Autodesk Inventor part; units mm, degrees
ref_plane "YZ Plane" through (0, 0, 0) normal (1, 0, 0) x (0, 1, 0)
ref_plane "XZ Plane" through (0, 0, 0) normal (0, 1, 0) x (-1, 0, 0)
ref_plane "XY Plane" through (0, 0, 0) normal (0, 0, 1) x (1, 0, 0)
sketch "Sketch1" plane through (0, 0, 0) normal (0, 0, 1) x (1, 0, 0)
  circle A0 centre (0, 0) radius 20
  line L0 (-85, -85) -> (85, -85)
  line L1 (85, -85) -> (85, 85)
  line L2 (85, 85) -> (-85, 85)
  line L3 (-85, 85) -> (-85, -85)
  line L4 (-85, -85) -> (85, 85) construction
  line L5 (85, -85) -> (-85, 85) construction
  dimension "d0" = 40
  dimension "d13" = 170
extrude "Extrusion1" add sketch "Sketch1" against normal blind 10
sketch "Sketch4" plane through (0, 0, 0) normal (0, 0, 1) x (1, 0, 0)
  line L0 (85, 85) -> (-85, 85)
  line L1 (-85, -85) -> (85, -85)
  line L2 (0, 0) -> (85, 85) construction
  circle A0 centre (65, 65) radius 6.5
  circle A1 centre (0, 0) radius 91.9239 construction
  dimension "d22" = 183.8478
  dimension "d23" = 13
  dimension "d24" = 65
  dimension "d25" = 65
extrude "Extrusion2" cut sketch "Sketch4" against normal through all
pattern_circular "Circular Pattern2" count 4 over 360 about axis through (0, 0, 0) along (0, 0, -1) of "Extrusion2"
fillet "Fillet1" radius 5 4 edges at (85, -85, -5) (-85, -85, -5) (-85, 85, -5) (85, 85, -5)
equation "\"BendReliefDepth\" = 0.5 * Thickness"
properties part number "NVPH-343 cup head flange"
Geometry: final body of the model. Coordinates: model frame, mm. Round coordinates to 2 decimals unless told otherwise and drop trailing zeros. Loops run counter-clockwise (first coordinate to the right, second up) from the corner with the lowest first, then second, coordinate; pieces in that order, holes last.
Q1. Pin query (flat end, axial travel): P1, Ø21, axis at x = 65, y = -65, coming from the -Z side. Return the tip coordinate at first contact, or that it passes through.
Q2. Section C-C on y = 0. Return loops of the section in (x, z), plus the area to 3 significant figures.
Q3. Material intervals for L1, parallel to Y at x = -65, z = -7; L2, parallel to Y at x = 0, z = -5.5, sorted ascending.
Q4. Pull-direction query (Y, two-part tool) for faces 1 (the flat face through (-20, 20, -10)), 2 (the cylindrical face through (-83, -84, -5)), 3 (the cylindrical face through (59.233, -67.999, -4.93)); classes: released by +Y, released by -Y, zero draft, split by the parting line, or undercut.
Q5. Section D-D on z = -1.5. Return loops of the section in (x, y).
Q6. Section A-A on x = 65. Return loops of the section in (y, z).
Evaluation:
1. P1: stops at z = -10
2. outline: (-85, -10) - (-20, -10) - (-20, 0) - (-85, 0) - close; (20, -10) - (85, -10) - (85, 0) - (20, 0) - close
2. area: 1,300 mm2
3. L1: y = -85 to -71.5, -58.5 to 58.5, 71.5 to 85
3. L2: y = -85 to -20, 20 to 85
4. face 1: zero draft
4. face 2: released by -Y
4. face 3: undercut
5. outline: (-85, -80) arc R5 ccw to (-80, -85) - (80, -85) arc R5 ccw to (85, -80) - (85, 80) arc R5 ccw to (80, 85) - (-80, 85) arc R5 ccw to (-85, 80) - close; hole circle Ø13 at (-65, -65); hole circle Ø13 at (-65, 65); hole circle Ø40 at (0, 0); hole circle Ø13 at (65, -65); hole circle Ø13 at (65, 65)
6. outline: (-85, -10) - (-71.5, -10) - (-71.5, 0) - (-85, 0) - close; (-58.5, -10) - (58.5, -10) - (58.5, 0) - (-58.5, 0) - close; (71.5, -10) - (85, -10) - (85, 0) - (71.5, 0) - close
